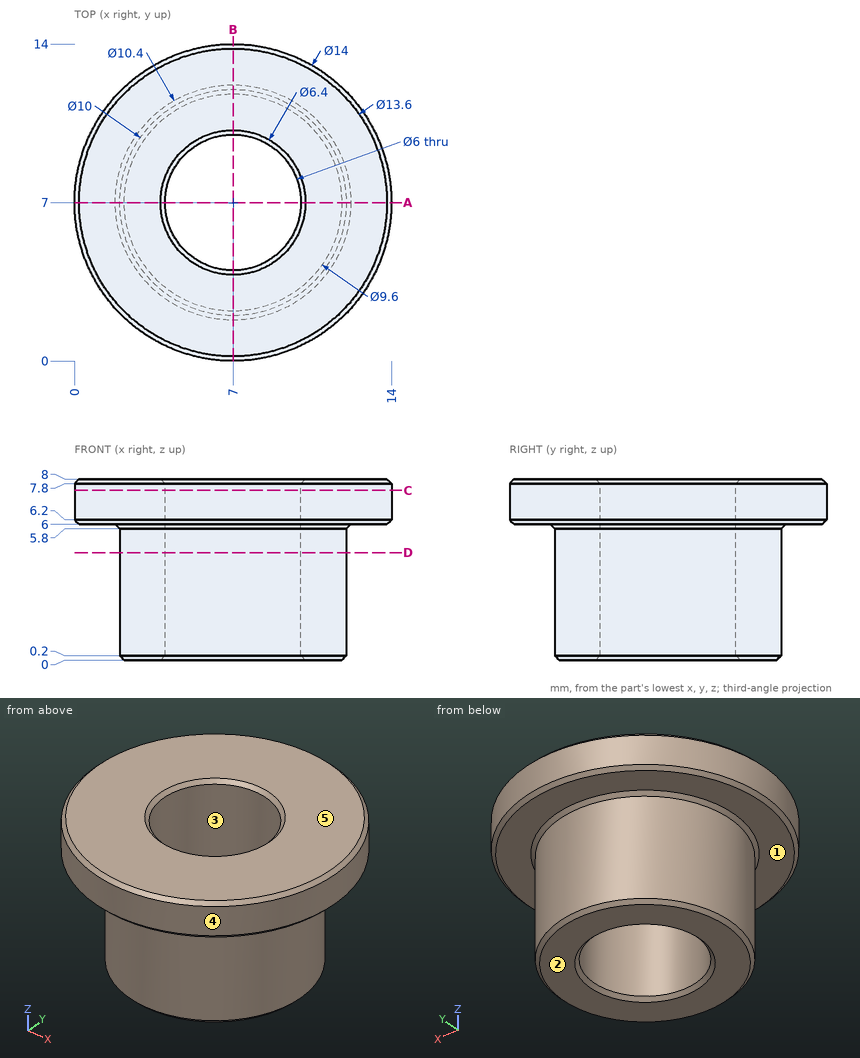
Source: three-view drawing plus pictorial views. Frame: mm from the lowest corner of the part. A direction names the side the tool comes from. Give positions to 0.01 mm unless a question says otherwise; leave off trailing zeros. Loops run counter-clockwise (first coordinate to the right, second up) from the corner with the lowest first, then second, coordinate; pieces in that order, holes last. Notation, with made-up numbers: (3, 87.25) -> (46, 87.25) arc R12 ccw to (46, 107.25) -> close; hole circle Ø1 at (3.5, 20.5). An arc over 180 degrees is marked (long way). Use a Markdown table: item, result. Add a question column.
(1) Section query D-D (z = 4.75). Output: boundary loops of the cut face in (x, y), then the cut area to 3 significant figures.
(2) Section query A-A (y = 7). Output: boundary loops of the cut face in (x, z).
(3) Pull-direction query (Y, two-part tool) for the marked faces 3, 4 and 5; classes: +Y half, -Y half, draft (parallel to the pull), parting line (faces both ways), or undercut.
(4) Access query for the marked faces 1 and 2. Directions: +Z, -Z, +X, -X, +Y, -Y. A direction counts if a zero-diameter tool reaches every point of the face in a straight line with its end or side. Return the directions, or none.
(5) First-contact query: pin 1 Ø1.5 at (x, z) = (9, 3) entering from +Y; pin 2 Ø1 at (y, z) = (2, 5) entering from -X; pin 3 Ø5.5 at (x, y) = (7, 7) entering from +Z. Flat tips, straight axial feed; report the tip coordinate or a pass-through.
(6) Section query C-C (z = 7.5). Output: boundary loops of the cut face in (x, y).
(7) Ray query, line 1 (Y direction, x = 7, z = 4.75); line 2 (X direction, y = 8, z = 1.75); line 3 (Z direction, x = 10, y = 12.5). Return the intervals inside material, ascending.
Checked values:
| question | item | result |
|---|---|---|
| 1 | outline | circle Ø10 at (7, 7); hole circle Ø6 at (7, 7) |
| 1 | area | 50.3 mm^2 |
| 2 | outline | (0, 6.2) -> (0.2, 6) -> (1.8, 6) -> (2, 5.8) -> (2, 0.2) -> (2.2, 0) -> (3.8, 0) -> (4, 0.2) -> (4, 7.8) -> (3.8, 8) -> (0.2, 8) -> (0, 7.8) -> close; (10, 0.2) -> (10.2, 0) -> (11.8, 0) -> (12, 0.2) -> (12, 5.8) -> (12.2, 6) -> (13.8, 6) -> (14, 6.2) -> (14, 7.8) -> (13.8, 8) -> (10.2, 8) -> (10, 7.8) -> close |
| 3 | face 3 | undercut |
| 3 | face 4 | parting line |
| 3 | face 5 | draft |
| 4 | face 1 | -Z |
| 4 | face 2 | -Z, +X, -X, +Y, -Y |
| 5 | pin 1 | y = 11.84 |
| 5 | pin 2 | x = 4.82 |
| 5 | pin 3 | through |
| 6 | outline | circle Ø14 at (7, 7); hole circle Ø6 at (7, 7) |
| 7 | line 1 | 2 to 4, 10 to 12 |
| 7 | line 2 | 2.1 to 4.17, 9.83 to 11.9 |
| 7 | line 3 | 6 to 8 |
